Check sheet for the modelled part. Datum: model origin and axes. Units: mm. Coordinates: 2 decimals unless noted, no trailing zeros. Order: outer loops, then holes, each group sorted by start corner. A loop starts at its lowest first (then second) coordinate and runs counter-clockwise, first axis right, second up.
1. Cross-section at C-C (y = -2.5). Enter the section's corners in (x, z), then the cut area to 3 significant figures.
2. Cross-section at B-B (z = -1.25). Enter the section's corners in (x, y).
3. Thickness scan on line 1 (X direction, y = -19.05, z = -4.9); line 2 (X direction, y = -5, z = -0.75); line 3 (Y direction, x = 42, z = -0.75). Record the ranges inside material, lowest first.
4. Draft check along X on faces 1 (the flat face through (66.253, -10, -3)), 2 (the cylindrical face through (63.148, -1.992, -3.219)), 3 (the flat face through (-1, -32.512, -3)). Enter one of: released by +X, released by -X, zero draft, split by the parting line, or undercut.
5. Cross-section at A-A (y = -19.05). Enter the section's corners in (x, z).
Autodesk Fusion 360 part; units mm, degrees
sketch "Sketch2" plane through (0, 0, 0) normal (0, 0, 1) x (1, 0, 0)
  line L0 (-66.2534, 12.7) -> (66.2534, 12.7)
  line L1 (66.2534, 12.7) -> (66.2534, -12.7)
  line L2 (66.2534, -12.7) -> (-66.2534, -12.7)
  line L3 (-66.2534, -12.7) -> (-66.2534, 12.7)
  line L4 (-66.2534, 0) -> (66.2534, 0) construction
  line L5 (0, 12.7) -> (0, -12.7) construction
  line L6 (-66.2534, -12.7) -> (66.2534, -12.7)
  line L7 (66.2534, -12.7) -> (66.2534, -32.512)
  line L8 (66.2534, -32.512) -> (-66.2534, -32.512)
  line L9 (-66.2534, -32.512) -> (-66.2534, -12.7)
  point P0 (-61.2521, 0)
  point P1 (61.2521, 0)
  point P2 (-40.8534, -19.05)
  point P3 (-61.2521, -3.2004)
  point P4 (61.2521, -3.2004)
  point P5 (40.8534, -19.05)
  dimension "d2" = 25.4
  dimension "d3" = 122.5042
  dimension "d4" = 132.5067
  dimension "d18" = 3.2004
  dimension "d19" = 25.4
  dimension "d22" = 19.05
  dimension "d23" = 19.812
extrude "Extrude1" add sketch "Sketch2" along normal blind 6.35
hole "Hole1" at (-61.2521, -3.2004, 0) at (61.2521, -3.2004, 0) direction (0, 0, 1) diameter 4.4958 end through all
hole "Hole2" at (-40.8534, -19.05, 0) at (40.8534, -19.05, 0) direction (0, 0, 1) diameter 4.4958 depth 7.62 tip angle 118 countersink diameter 8.4328 countersink angle 82
move_body "Move1" bodies 1 to x (-1, 0, 0) y (0, 1, 0) z (0, 0, -1) at (0, 0, 0)
equation "d3 = tiptop_spacing"
equation "d4 = 5.125 in + ( ( 0.0459 * 2 ) * 1 in )"
equation "synthrotek_spacing = 4.741 in"
equation "tiptop_spacing = 4.823 in"
Data:
1. outline: (-66.25, -6.35) - (-63.39, -6.35) - (-63.39, 0) - (-66.25, 0) - close; (-59.12, -6.35) - (59.12, -6.35) - (59.12, 0) - (-59.12, 0) - close; (63.39, -6.35) - (66.25, -6.35) - (66.25, 0) - (63.39, 0) - close
1. area: 787 mm2
2. outline: (-66.25, -32.51) - (66.25, -32.51) - (66.25, 12.7) - (-66.25, 12.7) - close; hole circle Ø4.5 at (-61.25, -3.2); hole circle Ø6.26 at (-40.85, -19.05); hole circle Ø6.26 at (40.85, -19.05); hole circle Ø4.5 at (61.25, -3.2)
3. line 1: x = -66.25 to -43.1, -38.61 to 38.61, 43.1 to 66.25
3. line 2: x = -66.25 to -62.6, -59.91 to 59.91, 62.6 to 66.25
3. line 3: y = -32.51 to -22.42, -15.68 to 12.7
4. face 1: released by +X
4. face 2: undercut
4. face 3: zero draft
5. outline: (-66.25, -6.35) - (-43.1, -6.35) - (-43.1, -2.26) - (-45.07, 0) - (-66.25, 0) - close; (-38.61, -6.35) - (38.61, -6.35) - (38.61, -2.26) - (36.64, 0) - (-36.64, 0) - (-38.61, -2.26) - close; (43.1, -6.35) - (66.25, -6.35) - (66.25, 0) - (45.07, 0) - (43.1, -2.26) - close
